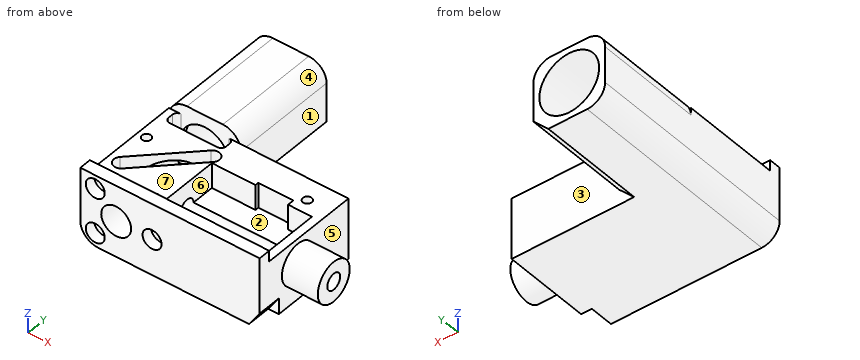
from build123d import *

# Parameters (mm, degrees)
SKETCH1_W                       = 15
SKETCH1_H                       = 6
MAIN_BODY_EXT_DEPTH             = 9.3
EMISSION_PATH_EXT_DEPTH         = 9
SKETCH3_R                       = 1.25
EMISSION_AND_GRIN_CUT_DEPTH     = 21.003499694
FIBER_FERRULE_CUT_REACH         = 25.851
FIBER_FERRULE_CUT_END_RADIUS    = 1.25
SKETCH4_R                       = 0.675
FIBER_START                     = 3
SKETCH41_R                      = 1.675
SKETCH41_R_2                    = 0.675
FIBER_FERRULE_PORT_EXT_DEPTH    = 3
SKETCH5_W                       = 15
SKETCH5_H                       = 8.3
FILTERSET_CUT1_DEPTH            = 0.9
FILTERSET_CUT2_DEPTH            = 4.2
SKETCH10_R                      = 2.5
EMISSION_LENS_CUT_DEPTH         = 8.5
EXCITATION_PATHWAY_CUT_2_DEPTH  = 2.1
SKETCH15_R                      = 0.795
MAGNETS_CUT_DEPTH               = 0.9
SCREW_HOLES_CUT_DEPTH           = 22.705990005
SCREW_HOLES_CUT_DEPTH_BACK      = 3
SKETCH18_R                      = 0.375
EXTERNAL_FILLET_1_R             = 1.5
EMISSION_PATHWAY_CUT_DEPTH      = 15.942891357
EMISSION_PATHWAY_CUT_DEPTH_BACK = 4
SKETCH28_R                      = 1.5
CUT_EXTRUDE16_DEPTH             = 9
CUT_EXTRUDE17_REACH             = 16.673
SKETCH37_R                      = 2
BASEPLATE_NOTCH_CUT_DEPTH       = 22.310560811
BASEPLATE_NOTCH_CUT_DEPTH_BACK  = 2


with BuildPart() as part:
    # Sketch1 → Main Body Ext (new body)
    with BuildSketch(Plane(origin=(0, 0, 0), x_dir=(1, 0, 0), z_dir=(0, 1, 0))):
        Rectangle(SKETCH1_W, SKETCH1_H)
    extrude(amount=MAIN_BODY_EXT_DEPTH)

    # Sketch8 → Emission Path Ext (add)
    with BuildSketch(Plane(origin=(0, 9.3, 0), x_dir=(1, 0, 0), z_dir=(0, 1, 0))):
        Polygon((-2.75, 3), (-1.5, 1.75), (-1.5, -3), (-7.5, -3), (-7.5, 3), align=None)
    extrude(amount=EMISSION_PATH_EXT_DEPTH)

    # Sketch3 → Emission and Grin Cut (cut, through all)
    with BuildSketch(Plane.XZ):
        with Locations(Location((-4.5, 0, 0), (0, 0, 270))):
            Circle(SKETCH3_R)
    extrude(amount=-EMISSION_AND_GRIN_CUT_DEPTH, mode=Mode.SUBTRACT)

    # Fiber Ferrule Cut: up to this cylinder (the profile starts outside it)
    fiber_ferrule_cut_end = Plane(origin=(-4.5, 4, 0), z_dir=(0, -1, 0)) * Cylinder(FIBER_FERRULE_CUT_END_RADIUS, 55.202, mode=Mode.PRIVATE)
    # Sketch4 → Fiber Ferrule Cut (cut, up to the surface)
    with BuildSketch(Plane(origin=(7.5, 0, 0), x_dir=(0, 0, -1), z_dir=(1, 0, 0)), mode=Mode.PRIVATE) as fiber_ferrule_cut_sk1:
        with Locations((0, 4)):
            Circle(SKETCH4_R)
    fiber_ferrule_cut_tool1 = extrude(fiber_ferrule_cut_sk1.sketch, amount=-FIBER_FERRULE_CUT_REACH, mode=Mode.PRIVATE) - fiber_ferrule_cut_end
    add(fiber_ferrule_cut_tool1.solids().sort_by_distance((7.5, 4, 0))[0], mode=Mode.SUBTRACT)

    # Sketch41 → Fiber Ferrule Port Ext (add)
    with BuildSketch(Plane(origin=(7.5, 0, 0), x_dir=(0, 0, -1), z_dir=(1, 0, 0)).offset(FIBER_START)):
        with Locations(Location((0, 4, 0), (0, 0, 180))):
            Circle(SKETCH41_R)
        with Locations((0, 4)):
            Circle(SKETCH41_R_2, mode=Mode.SUBTRACT)
    extrude(amount=-FIBER_FERRULE_PORT_EXT_DEPTH)

    # Sketch5 → FilterSet Cut1 (cut)
    with BuildSketch(Plane.XY.offset(3)):
        with Locations((0, 5.15)):
            Rectangle(SKETCH5_W, SKETCH5_H)
    extrude(amount=-FILTERSET_CUT1_DEPTH, mode=Mode.SUBTRACT)

    # Sketch6 → FilterSet Cut2 (cut)
    with BuildSketch(Plane.XY.offset(2.1)):
        with BuildLine():
            Line((-2.60588745, 7.591168825), (-6.848528137, 3.348528137))
            ThreePointArc((-6.848528137, 3.348528137), (-6.848528137, 2.5), (-6, 2.5))
            Line((-6, 2.5), (-1.757359313, 6.742640687))
            ThreePointArc((-1.757359313, 6.742640687), (-1.757359313, 7.591168825), (-2.60588745, 7.591168825))
        make_face()
        with BuildLine():
            ThreePointArc((-6.5, 9.3), (-6.782842712, 9.182842712), (-6.9, 8.9))
            Line((-6.9, 8.9), (-6.9, 8.5))
            ThreePointArc((-6.9, 8.5), (-6.782842712, 8.217157288), (-6.5, 8.1))
            Line((-6.5, 8.1), (-2.5, 8.1))
            ThreePointArc((-2.5, 8.1), (-2.217157288, 8.217157288), (-2.1, 8.5))
            Line((-2.1, 8.5), (-2.1, 8.9))
            ThreePointArc((-2.1, 8.9), (-2.217157288, 9.182842712), (-2.5, 9.3))
            Line((-2.5, 9.3), (-6.5, 9.3))
        make_face()
    extrude(amount=-FILTERSET_CUT2_DEPTH, mode=Mode.SUBTRACT)

    # Sketch10 → Emission Lens Cut (cut)
    with BuildSketch(Plane(origin=(0, 18.3, 0), x_dir=(1, 0, 0), z_dir=(0, 1, 0))):
        with Locations(Location((-4.5, 0, 0), (0, 0, 270))):
            Circle(SKETCH10_R)
    extrude(amount=-EMISSION_LENS_CUT_DEPTH, mode=Mode.SUBTRACT)

    # Sketch44 → Excitation Pathway Cut 2 (cut)
    with BuildSketch(Plane.XY):
        Polygon((3.4, 1.1), (1.88, 1.1), (1.88, 1.4), (0.6, 1.4), (-0.9, 1.4), (-1.76, 1.4), (-1.76, 6.6), (-0.9, 6.6), (0.6, 6.6), (1.88, 6.6), (1.88, 6.9), (3.4, 6.9), (4.81, 6.9), (4.81, 6.35), (6.81, 6.35), (6.81, 1.65), (4.81, 1.65), (4.81, 1.1), align=None)
    extrude(amount=EXCITATION_PATHWAY_CUT_2_DEPTH, mode=Mode.SUBTRACT)

    # Sketch15 → Magnets Cut (cut)
    with BuildSketch(Plane.XZ):
        with Locations(Location((-6.25, -1.875, 0), (0, 0, 270))):
            Circle(SKETCH15_R)
        with Locations(Location((-6.25, 1.875, 0), (0, 0, 270))):
            Circle(SKETCH15_R)
        with Locations(Location((-1.5, 0, 0), (0, 0, 270))):
            Circle(SKETCH15_R)
    extrude(amount=-MAGNETS_CUT_DEPTH, mode=Mode.SUBTRACT)

    # Sketch18 → Screw Holes Cut (cut, two sides: drawn at the far end of the back side and taken through both)
    with BuildSketch(Plane.XY.offset(2.1).offset(-SCREW_HOLES_CUT_DEPTH_BACK)):
        with Locations(Location((-6.75, 6, 0), (0, 0, 180))):
            Circle(SKETCH18_R)
        with Locations(Location((5.5, 7.5, 0), (0, 0, 180))):
            Circle(SKETCH18_R)
        with Locations(Location((-2.5, 1.51, 0), (0, 0, 180))):
            Circle(SKETCH18_R)
    extrude(amount=SCREW_HOLES_CUT_DEPTH + SCREW_HOLES_CUT_DEPTH_BACK, mode=Mode.SUBTRACT)

    # External Fillet 1
    # the kernel refuses this fillet: 1.5 mm, written as the material it takes off along each edge
    with BuildSketch(Plane(origin=(-7.5, -3.75, -3), x_dir=(1, 0, 0), z_dir=(0, 1, 0))) as external_fillet_1_piece_1:
        with BuildLine():
            CenterArc((EXTERNAL_FILLET_1_R, -EXTERNAL_FILLET_1_R), EXTERNAL_FILLET_1_R, 90, 90)
            Line((0, -EXTERNAL_FILLET_1_R), (0, 0))
            Line((0, 0), (EXTERNAL_FILLET_1_R, 0))
        make_face()
    extrude(amount=25.8, mode=Mode.SUBTRACT)
    with BuildSketch(Plane(origin=(-1.5, 9.3, 3), x_dir=(0, 0, -1), z_dir=(0, 1, 0))) as external_fillet_1_piece_2:
        with BuildLine():
            CenterArc((EXTERNAL_FILLET_1_R, EXTERNAL_FILLET_1_R), EXTERNAL_FILLET_1_R, 180, 90)
            Line((0, EXTERNAL_FILLET_1_R), (0, 0))
            Line((0, 0), (EXTERNAL_FILLET_1_R, 0))
        make_face()
    extrude(amount=12.75, mode=Mode.SUBTRACT)

    # Sketch28 → Emission Pathway Cut (cut, two sides: drawn at the far end of the back side and taken through both)
    with BuildSketch(Plane(origin=(0, 8.1, 0), x_dir=(1, 0, 0), z_dir=(0, 1, 0)).offset(-EMISSION_PATHWAY_CUT_DEPTH_BACK)):
        with Locations(Location((-4.5, 0, 0), (0, 0, 180))):
            Circle(SKETCH28_R)
    extrude(amount=EMISSION_PATHWAY_CUT_DEPTH + EMISSION_PATHWAY_CUT_DEPTH_BACK, mode=Mode.SUBTRACT)

    # Sketch36 → Cut-Extrude16 (cut)
    with BuildSketch(Plane(origin=(0, 18.3, 0), x_dir=(1, 0, 0), z_dir=(0, 1, 0))):
        with BuildLine():
            Line((-7.5, -1.5), (-7.5, -3))
            Line((-7.5, -3), (-6, -3))
            ThreePointArc((-6, -3), (-7.060660172, -2.560660172), (-7.5, -1.5))
        make_face()
    extrude(amount=-CUT_EXTRUDE16_DEPTH, mode=Mode.SUBTRACT)

    # Sketch37 → Cut-Extrude17 (cut, up to next)
    with BuildSketch(Plane(origin=(0, 9.8, 0), x_dir=(1, 0, 0), z_dir=(0, 1, 0)), mode=Mode.PRIVATE) as cut_extrude17_sk1:
        with Locations(Location((-4.5, 0, 0), (0, 0, 180))):
            Circle(SKETCH37_R)
    cut_extrude17_tool1 = extrude(cut_extrude17_sk1.sketch, amount=-CUT_EXTRUDE17_REACH, mode=Mode.PRIVATE) & part.part
    add(cut_extrude17_tool1.solids().sort_by_distance((-4.5, 9.8, 0))[0], mode=Mode.SUBTRACT)

    # Sketch45 → Baseplate Notch Cut (cut, two sides: drawn at the far end of the back side and taken through both)
    with BuildSketch(Plane.XZ.offset(-BASEPLATE_NOTCH_CUT_DEPTH_BACK)):
        Polygon((30.47380128, 32.796887648), (7.5, -1.663902268), (6.609270453, -3), (-16.364530827, -37.460789916), (52.557049005, -83.408392475), (99.395381111, -13.150714911), align=None)
    extrude(amount=BASEPLATE_NOTCH_CUT_DEPTH + BASEPLATE_NOTCH_CUT_DEPTH_BACK, mode=Mode.SUBTRACT)


solid = part.part
Geometry: final body of the model. Coordinates: model frame, mm. Face numbers are marked on the shaded views. A direction names the side the tool comes from. Give positions to 0.01 mm unless a question says otherwise; leave off trailing zeros. Write each loop counter-clockwise with the first axis right and the second up, starting at its lowest first coordinate (ties: lowest second). Pieces come first, ordered by that corner, then holes. Notation, with made-up numbers: (22.25, -38) - (70.25, -38) arc R22 ccw to (70.25, -13) - close; hole circle Ø8 at (-2.75, -36.75). An arc over 180 degrees is marked (long way). Return JSON: item names as keys, results as strings. Group by question number.
1) Section B-B on x = 0.5. Return the cut outline in (y, z) (3 decimals), plus the area to 3 significant figures.
2) Set-up query: the marked faces 4, 5, 6 and 7. Return all of +Z, -Z, +X, -X, +Y, -Y with unobstructed straight access to the full face (end or side cutting, diameter ignored); none if empty.
3) Section A-A on y = 14. Return the cut outline in (x, z).
4) Section D-D on x = 8.25. Return the cut outline in (y, z) (3 decimals), plus the area to 3 significant figures.
5) Section C-C on y = 5.25. Return the cut outline in (x, z), plus the area to 3 significant figures.
6) First-contact query: P1, Ø1, axis at x = 5.5, z = 1, coming from the +Y side; P2, Ø1, axis at x = -5.5, y = 8.5, coming from the +Z side; P3, Ø0.7, axis at x = 1.5, y = 6, coming from the +Z side. Flat tips, straight axial feed; report the tip coordinate or a pass-through.
7) Line query: line 1 (X direction, y = 2.75, z = 2); line 2 (X direction, y = 14.25, z = 1.5); line 3 (Y direction, x = -2.5, z = 0.6) (3 decimals). Output: solid intervals per line, ascending.
8) Mould query, pull axis X, two halves, no side actions, for the marked faces 1, 2 and 3. Classes: released by +X, released by -X, zero draft, split by the parting line, or undercut.
Filled in:
{
 "1": {"outline": "(0, -3) - (9.3, -3) - (9.3, 2.1) - (6.6, 2.1) - (6.6, 0) - (4.675, 0) arc R0.675 cw to (3.325, 0) - (1.4, 0) - (1.4, 2.1) - (1, 2.1) - (1, 3) - (0, 3) - close", "area": "36.7 mm^2"},
 "2": {"face 4": "+Z, +X, +Y", "face 5": "+X", "face 6": "+Z", "face 7": "+Z, +X, -X"},
 "3": {"outline": "(-7.5, -1.5) arc R1.5 ccw to (-6, -3) - (-2.75, -3) - (-1.5, -1.75) - (-1.5, 1.5) arc R1.5 ccw to (-3, 3) - (-6, 3) arc R1.5 ccw to (-7.5, 1.5) - close; hole circle Ø5 at (-4.5, 0)"},
 "4": {"outline": "circle Ø3.35 at (4, 0); hole circle Ø1.35 at (4, 0)", "area": "7.38 mm^2"},
 "5": {"outline": "(-7.5, -1.5) arc R1.5 ccw to (-6, -3) - (7.5, -3) - (7.5, -1.11) - (10.5, -1.11) - (10.5, 1.11) - (7.5, 1.11) - (7.5, 2.1) - (6.81, 2.1) - (6.81, 0) - (-1.76, 0) - (-1.76, 2.1) - (-3.25, 2.1) - (-3.25, 0.83) arc R1.5 cw to (-3.25, -0.83) - (-3.25, -2.1) - (-4.95, -2.1) - (-4.95, -1.43) arc R1.5 cw to (-4.95, 1.43) - (-4.95, 2.1) - (-7.5, 2.1) - close", "area": "55.1 mm^2"},
 "6": {"P1": "stops at y = 9.3", "P2": "stops at z = 2.1", "P3": "stops at z = 0"},
 "7": {"line 1": "x = -7.5 to -7, -5.75 to -1.76, 6.81 to 7.5", "line 2": "x = -7.5 to -6.5, -2.5 to -1.5", "line 3": "y = 0 to 1.135, 1.885 to 3.691, 4.309 to 6, 7.675 to 8.1, 9.3 to 9.8"},
 "8": {"face 1": "released by +X", "face 2": "undercut", "face 3": "zero draft"}
}
